from build123d import *

# Parameters (mm, degrees)
BOSS_EXTRUDE1_DEPTH = 17.5
SKETCH2_R           = 1.6
CUT_EXTRUDE1_DEPTH  = 4.41
SKETCH3_R           = 2.75
CUT_EXTRUDE2_DEPTH  = 1.2
SKETCH4_W           = 8.58
SKETCH4_H           = 35
CUT_EXTRUDE3_DEPTH  = 0.6
FILLET1_R           = 0.6


with BuildPart() as part:
    # Sketch1 → Boss-Extrude1 (new body, symmetric)
    with BuildSketch(Plane.XY):
        with BuildLine():
            Line((-3.14, 0.055), (-3.14, -0.055))
            ThreePointArc((-3.14, -0.055), (-3.476827202, -0.868172798), (-4.29, -1.205))
            Line((-4.29, -1.205), (-4.29, -1.705))
            Line((-4.29, -1.705), (4.29, -1.705))
            Line((4.29, -1.705), (4.29, -1.205))
            ThreePointArc((4.29, -1.205), (3.476827202, -0.868172798), (3.14, -0.055))
            Line((3.14, -0.055), (3.14, 0.055))
            ThreePointArc((3.14, 0.055), (3.476827202, 0.868172798), (4.29, 1.205))
            Line((4.29, 1.205), (4.29, 1.705))
            Line((4.29, 1.705), (-4.29, 1.705))
            Line((-4.29, 1.705), (-4.29, 1.205))
            ThreePointArc((-4.29, 1.205), (-3.476827202, 0.868172798), (-3.14, 0.055))
        make_face()
    extrude(amount=BOSS_EXTRUDE1_DEPTH, both=True)

    # Sketch2 → Cut-Extrude1 (cut, through all)
    with BuildSketch(Plane(origin=(0, 1.705, 0), x_dir=(1, 0, 0), z_dir=(0, 1, 0))):
        with Locations((0, 12.5)):
            Circle(SKETCH2_R)
    cut_extrude1 = extrude(amount=-CUT_EXTRUDE1_DEPTH, mode=Mode.SUBTRACT)

    # Sketch3 → Cut-Extrude2 (cut)
    with BuildSketch(Plane(origin=(0, 1.705, 0), x_dir=(1, 0, 0), z_dir=(0, 1, 0))):
        with Locations((0, 12.5)):
            Circle(SKETCH3_R)
    cut_extrude2 = extrude(amount=-CUT_EXTRUDE2_DEPTH, mode=Mode.SUBTRACT)

    # Mirror1: Cut-Extrude1, Cut-Extrude2 across plane
    add(cut_extrude1.mirror(Plane.XY), mode=Mode.SUBTRACT)
    add(cut_extrude2.mirror(Plane.XY), mode=Mode.SUBTRACT)

    # Sketch4 → Cut-Extrude3 (cut)
    with BuildSketch(Plane.XZ.offset(1.705)):
        Rectangle(SKETCH4_W, SKETCH4_H)
    extrude(amount=-CUT_EXTRUDE3_DEPTH, mode=Mode.SUBTRACT)

    # Fillet1
    fillet1_edges = [part.edges().sort_by_distance(p)[0] for p in [
        (0, 1.705, -17.5),
        (0, 1.705, 17.5),
    ]]
    fillet(fillet1_edges, radius=FILLET1_R)


solid = part.part
Design review of the part built by this model. Coordinates are the model's own, in mm. A direction names the side the tool comes from. Round coordinates to 2 decimals unless told otherwise and drop trailing zeros. Write each loop counter-clockwise with the first axis right and the second up, starting at its lowest first coordinate (ties: lowest second). Pieces come first, ordered by that corner, then holes. Notation, with made-up numbers: (-21, -7.5) -> (13, -7.5) arc R6 ccw to (13, 3.5) -> close; hole circle Ø11 at (53, 40.25). An arc over 180 degrees is marked (long way). One line per question, with ' | ' between items.
(1) Insertion check: P1, Ø1.9, axis at x = 0, z = -12.5, coming from the -Y side; P2, Ø4.5, axis at x = 0, z = 12.5, coming from the +Y side (3 decimals). Each pin has a flat end and moves straight along its axis. Give the tip position at first contact, or say it passes through.
Result sheet:
P1: through | P2: y = 0.505
(2) Take a section at A-A, the plane x = 0. State the section outline as (y, z) points (3 decimals).
Result sheet:
outline: (-1.105, -17.5) -> (1.105, -17.5) arc R0.6 ccw to (1.705, -16.9) -> (1.705, -15.25) -> (0.505, -15.25) -> (0.505, -14.1) -> (-1.105, -14.1) -> close; (-1.105, -10.9) -> (0.505, -10.9) -> (0.505, -9.75) -> (1.705, -9.75) -> (1.705, 9.75) -> (0.505, 9.75) -> (0.505, 10.9) -> (-1.105, 10.9) -> close; (-1.105, 14.1) -> (0.505, 14.1) -> (0.505, 15.25) -> (1.705, 15.25) -> (1.705, 16.9) arc R0.6 ccw to (1.105, 17.5) -> (-1.105, 17.5) -> close
(3) Wall thickness on line 1 (Z direction, x = -1, y = -0.2); line 2 (Z direction, x = 0, y = 1.3); line 3 (X direction, y = 0, z = 12.5): over which ranges is each line inside the solid? List them lowest first. Write a range as [from, to].
Result sheet:
line 1: [-17.5, -13.75], [-11.25, 11.25], [13.75, 17.5] | line 2: [-17.47, -15.25], [-9.75, 9.75], [15.25, 17.47] | line 3: [-3.14, -1.6], [1.6, 3.14]
(4) Take a section at D-D, the plane z = 2.5. State the section outline as (x, y) points (3 decimals), and give its area (3 significant figures).
Result sheet:
outline: (-4.29, 1.205) arc R1.15 cw to (-3.14, 0.055) -> (-3.14, -0.055) arc R1.15 cw to (-3.821, -1.105) -> (3.821, -1.105) arc R1.15 cw to (3.14, -0.055) -> (3.14, 0.055) arc R1.15 cw to (4.29, 1.205) -> (4.29, 1.705) -> (-4.29, 1.705) -> close | area: 19.8 mm2
(5) Take a section at C-C, the plane x = -3.5. State the section outline as (y, z) points (3 decimals), and give its area (3 significant figures).
Result sheet:
outline: (-1.105, -17.5) -> (-0.891, -17.5) -> (-0.891, 17.5) -> (-1.105, 17.5) -> close; (0.891, -17.5) -> (1.105, -17.5) arc R0.6 ccw to (1.705, -16.9) -> (1.705, 16.9) arc R0.6 ccw to (1.105, 17.5) -> (0.891, 17.5) -> close | area: 35.8 mm2
(6) Draft analysis for pull direction X (two halves, no side actions). For faces 5 (the cylindrical face through (3.47, 0.86, 0.25)), 6 (the flat face through (1, 0.505, 11)), 7 (the flat face through (0, 0, 17.5)), state which applies: released by +X, released by -X, zero draft, split by the parting line, or undercut.
Result sheet:
face 5: released by +X | face 6: undercut | face 7: zero draft
(7) Machinability: for faces 1 (the cylindrical face through (3.33, -0.69, 0.25)), 2 (the flat face through (0, 1.705, 0)), 3 (the cylindrical face through (-3.32, -0.67, 0.25)), 4 (the flat face through (1, 0.505, -11)), which of the approach directions +Z, -Z, +X, -X, +Y, -Y give a long, thin tool a straight path to every point of the face, cutting with its end or side? Answer none if there is none.
Result sheet:
face 1: +Z, -Z, +X | face 2: +Z, -Z, +X, -X, +Y | face 3: +Z, -Z, -X | face 4: +Y
(8) Take a section at B-B, the plane z = 12.5. State the section outline as (x, y) points (3 decimals).
Result sheet:
outline: (-4.29, 1.205) arc R1.15 cw to (-3.14, 0.055) -> (-3.14, -0.055) arc R1.15 cw to (-3.821, -1.105) -> (-1.6, -1.105) -> (-1.6, 0.505) -> (-2.75, 0.505) -> (-2.75, 1.705) -> (-4.29, 1.705) -> close; (1.6, -1.105) -> (3.821, -1.105) arc R1.15 cw to (3.14, -0.055) -> (3.14, 0.055) arc R1.15 cw to (4.29, 1.205) -> (4.29, 1.705) -> (2.75, 1.705) -> (2.75, 0.505) -> (1.6, 0.505) -> close
